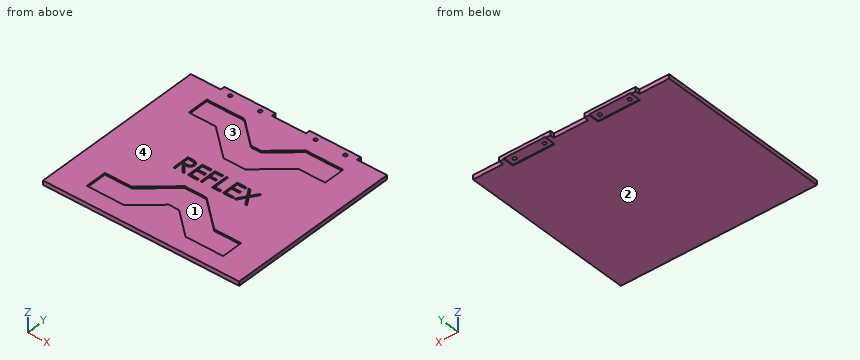
```python
from build123d import *

# Parameters (mm, degrees)
BOSS_EXTRU_1_DEPTH      = 5
ENL_V_MAT_EXTRU_2_DEPTH = 2
ENL_V_MAT_EXTRU_3_DEPTH = 2
ESQUISSE4_W             = 49
ESQUISSE4_H             = 12.519470299
ENL_V_MAT_EXTRU_5_DEPTH = 1
ESQUISSE5_R             = 2
ENL_V_MAT_EXTRU_6_DEPTH = 262.315639817


with BuildPart() as part:
    # Esquisse1 → Boss.-Extru.1 (new body)
    with BuildSketch(Plane.XY):
        Polygon((-56, 10.102941176), (-21, 10.102941176), (-21, 15.102941176), (39, 15.102941176), (39, 10.102941176), (79, 10.102941176), (79, 15.102941176), (139, 15.102941176), (139, 10.102941176), (174, 10.102941176), (174, -194.897058824), (-56, -194.897058824), align=None)
    extrude(amount=BOSS_EXTRU_1_DEPTH)

    # Esquisse2 → Enlèv. mat.-Extru.2 (cut)
    with BuildSketch(Plane.XY.offset(5)):
        Polygon((23.144921781, -9.214330656), (-20.950579999, -9.214330656), (-20.950579999, -34.214330656), (10.659241187, -34.214330656), (46.203012632, -65.443309996), (71.796987368, -65.443309996), (107.340758813, -34.214330656), (138.950579999, -34.214330656), (138.950579999, -9.214330656), (94.855078219, -9.214330656), (65.002138205, -35.443309996), (52.997861795, -35.443309996), align=None)
        Polygon((10.659241187, -150.579786991), (-20.950579999, -150.579786991), (-20.950579999, -175.579786991), (23.144921781, -175.579786991), (52.997861795, -149.350807651), (65.002138205, -149.350807651), (94.855078219, -175.579786991), (138.950579999, -175.579786991), (138.950579999, -150.579786991), (107.340758813, -150.579786991), (71.796987368, -119.350807651), (46.203012632, -119.350807651), align=None)
    extrude(amount=-ENL_V_MAT_EXTRU_2_DEPTH, mode=Mode.SUBTRACT)

    # Esquisse3 → Enlèv. mat.-Extru.3 (cut)
    # profile 1 of 6: a face of its own
    with BuildSketch(Plane.XY.offset(5)):
        with BuildLine():
            Line((20.856664396, -84.979311094), (24.859068242, -84.979311094))
            add(Edge.make_bspline(
                [(24.859068242, -84.979311094), (25.126160405, -84.980200157), (25.639006945, -84.981907256), (26.373711347, -84.991425901), (27.041294758, -85.018707934), (27.641408126, -85.042185554), (28.17404044, -85.084996647), (28.640824959, -85.125914631), (29.039611801, -85.179478407), (29.281016666, -85.229223681), (29.390318242, -85.251746992)],
                knots=[0, 0, 0, 0, 1.410062039, 2.707475311, 3.878576406, 4.937260626, 5.877586885, 6.699081471, 7.410979367, 8, 8, 8, 8], degree=3))
            add(Edge.make_bspline(
                [(29.390318242, -85.251746992), (29.536641809, -85.287899937), (29.826167463, -85.359434586), (30.243024983, -85.510632305), (30.640249692, -85.685601589), (31.016191545, -85.891108562), (31.368967495, -86.128678732), (31.702214985, -86.39421086), (32.017446204, -86.686252036), (32.301912662, -87.012165416), (32.570135815, -87.354088328), (32.796356538, -87.723824081), (32.991364993, -88.110461382), (33.14662509, -88.51793234), (33.271642082, -88.942285322), (33.359792021, -89.387364161), (33.41265595, -89.851141161), (33.418037982, -90.167472069), (33.42076696, -90.327868787)],
                knots=[0, 0, 0, 0, 1.027469482, 2.033020251, 3.019912614, 3.986113645, 4.951240523, 5.91722682, 6.890402269, 7.87763091, 8.8651537, 9.85103654, 10.82876324, 11.815024772, 12.821070561, 13.842952187, 14.906261191, 16, 16, 16, 16], degree=3))
            add(Edge.make_bspline(
                [(33.42076696, -90.327868787), (33.412372686, -90.594355099), (33.395993281, -91.114338915), (33.243278403, -91.868972523), (32.993126862, -92.572911464), (32.648422353, -93.225269395), (32.20945392, -93.813330226), (31.681883685, -94.329847113), (31.065417334, -94.762075185), (30.491535529, -95.061805498), (29.984597245, -95.253764975), (29.567264029, -95.388829883), (29.112024157, -95.493183971), (28.623239388, -95.586670438), (28.098875642, -95.657251549), (27.540189703, -95.708946374), (26.946783122, -95.741255224), (26.539131297, -95.74606668), (26.329420807, -95.748541864)],
                knots=[0, 0, 0, 0, 1.260483769, 2.459530307, 3.627416485, 4.787058657, 5.939039949, 7.08810263, 8.267026773, 9.491475466, 10.141966685, 10.831826277, 11.566392101, 12.351337768, 13.187381173, 14.07005841, 15.007169909, 16, 16, 16, 16], degree=3))
            Line((26.329420807, -95.748541864), (33.677177217, -104.979311094))
            Line((33.677177217, -104.979311094), (31.457625935, -104.979311094))
            Line((31.457625935, -104.979311094), (24.109869525, -95.748541864))
            Line((24.109869525, -95.748541864), (22.651536191, -95.748541864))
            Line((22.651536191, -95.748541864), (22.651536191, -104.979311094))
            Line((22.651536191, -104.979311094), (20.856664396, -104.979311094))
            Line((20.856664396, -104.979311094), (20.856664396, -84.979311094))
        make_face()
        with BuildLine():
            Line((22.651536191, -87.030593146), (22.651536191, -93.697259812))
            Line((22.651536191, -93.697259812), (26.313395166, -93.725304684))
            add(Edge.make_bspline(
                [(26.313395166, -93.725304684), (26.484366817, -93.725380322), (26.815758571, -93.72552693), (27.295190942, -93.702705352), (27.74159158, -93.676743533), (28.153253021, -93.637032987), (28.530359166, -93.585855434), (28.872721527, -93.521838382), (29.180898966, -93.447255167), (29.540319186, -93.331817305), (29.941670794, -93.148925772), (30.377850564, -92.882837208), (30.749292494, -92.548156527), (31.06310885, -92.165451064), (31.31527703, -91.744672499), (31.493060198, -91.290864675), (31.605874154, -90.815484115), (31.619180128, -90.48875207), (31.625895166, -90.323862376)],
                knots=[0, 0, 0, 0, 1.146690395, 2.22261258, 3.21895312, 4.145990853, 4.996080663, 5.770904154, 6.481378293, 7.121626537, 8.300444488, 9.431385265, 10.535395872, 11.636531494, 12.74115979, 13.810798291, 14.895190096, 16, 16, 16, 16], degree=3))
            add(Edge.make_bspline(
                [(31.625895166, -90.323862376), (31.619025902, -90.163024812), (31.605413529, -89.844303448), (31.494277709, -89.377698247), (31.306338387, -88.937315675), (31.053068456, -88.524947189), (30.744501856, -88.150628698), (30.382685783, -87.830359252), (29.977513239, -87.566076597), (29.598820677, -87.397194423), (29.260339463, -87.293652404), (28.966455692, -87.220788611), (28.634390105, -87.162248788), (28.262530341, -87.115345583), (27.852463879, -87.075031616), (27.402117302, -87.047878595), (26.914478557, -87.031799372), (26.576496094, -87.031004578), (26.401536191, -87.030593146)],
                knots=[0, 0, 0, 0, 1.101028733, 2.181837193, 3.264309656, 4.369019818, 5.486613113, 6.575447106, 7.666700264, 8.788928104, 9.402425223, 10.0903467, 10.862060571, 11.710948788, 12.657782767, 13.684531032, 14.801375019, 16, 16, 16, 16], degree=3))
            Line((26.401536191, -87.030593146), (22.651536191, -87.030593146))
        make_face(mode=Mode.SUBTRACT)
    # profile 2 of 6: a face of its own
    with BuildSketch(Plane.XY.offset(5)):
        Polygon((37.779741319, -84.979311094), (49.061792601, -84.979311094), (49.061792601, -87.030593146), (39.574613114, -87.030593146), (39.574613114, -93.184439299), (49.061792601, -93.184439299), (49.061792601, -95.235721351), (39.574613114, -95.235721351), (39.574613114, -102.928029043), (49.061792601, -102.928029043), (49.061792601, -104.979311094), (37.779741319, -104.979311094), align=None)
    # profile 3 of 6: a face of its own
    with BuildSketch(Plane.XY.offset(5)):
        Polygon((52.651536191, -84.979311094), (62.395125935, -84.979311094), (62.395125935, -87.030593146), (54.446407986, -87.030593146), (54.446407986, -93.184439299), (62.395125935, -93.184439299), (62.395125935, -95.235721351), (54.446407986, -95.235721351), (54.446407986, -104.979311094), (52.651536191, -104.979311094), align=None)
    # profile 4 of 6: a face of its own
    with BuildSketch(Plane.XY.offset(5)):
        Polygon((65.984869525, -84.979311094), (67.779741319, -84.979311094), (67.779741319, -102.928029043), (75.472049012, -102.928029043), (75.472049012, -104.979311094), (65.984869525, -104.979311094), align=None)
    # profile 5 of 6: a face of its own
    with BuildSketch(Plane.XY.offset(5)):
        Polygon((78.805382345, -84.979311094), (90.087433627, -84.979311094), (90.087433627, -87.030593146), (80.60025414, -87.030593146), (80.60025414, -93.184439299), (90.087433627, -93.184439299), (90.087433627, -95.235721351), (80.60025414, -95.235721351), (80.60025414, -102.928029043), (90.087433627, -102.928029043), (90.087433627, -104.979311094), (78.805382345, -104.979311094), align=None)
    # profile 6 of 6: a face of its own
    with BuildSketch(Plane.XY.offset(5)):
        Polygon((92.266920807, -84.979311094), (94.338234909, -84.979311094), (99.574613114, -93.160400838), (104.810991319, -84.979311094), (106.882305422, -84.979311094), (100.612273371, -94.778990582), (107.138715678, -104.979311094), (105.067401576, -104.979311094), (99.574613114, -96.397580325), (94.081824653, -104.979311094), (92.01051055, -104.979311094), (98.540959268, -94.778990582), align=None)
    extrude(amount=-ENL_V_MAT_EXTRU_3_DEPTH, mode=Mode.SUBTRACT)

    # Esquisse4 → Enlèv. mat.-Extru.5 (cut)
    with BuildSketch(Plane(origin=(0, 0, 0), x_dir=(-1, 0, 0), z_dir=(0, 0, -1))):
        with Locations((-9, 8.843206027)):
            Rectangle(ESQUISSE4_W, ESQUISSE4_H)
        with Locations((-109, 8.843206027)):
            Rectangle(ESQUISSE4_W, ESQUISSE4_H)
    extrude(amount=-ENL_V_MAT_EXTRU_5_DEPTH, mode=Mode.SUBTRACT)

    # Esquisse5 → Enlèv. mat.-Extru.6 (cut, through all)
    with BuildSketch(Plane(origin=(0, 0, 0), x_dir=(-1, 0, 0), z_dir=(0, 0, -1))):
        with Locations((8.5, 8.583470877)):
            Circle(ESQUISSE5_R)
        with Locations(Location((-26.5, 8.583470877, 0), (0, 0, 180))):
            Circle(ESQUISSE5_R)
        with Locations((-126.5, 8.583470877)):
            Circle(ESQUISSE5_R)
        with Locations((-91.5, 8.583470877)):
            Circle(ESQUISSE5_R)
    extrude(amount=-ENL_V_MAT_EXTRU_6_DEPTH, mode=Mode.SUBTRACT)


solid = part.part
```
The model under review builds one solid part; all positions refer to its coordinate system, in mm. Face numbers are marked on the shaded views. A direction names the side the tool comes from. Round coordinates to 2 decimals unless told otherwise and drop trailing zeros. Write each loop counter-clockwise with the first axis right and the second up, starting at its lowest first coordinate (ties: lowest second). Pieces come first, ordered by that corner, then holes.
(1) We need section A-A on x = 4. Give the boundary of the cut face in (y, z).
(2) We need section C-C on y = -134. Give the boundary of the cut face in (x, z), and give its area (3 significant figures).
(3) Insertion check: pin 1 (2 mm diameter, centred on x = 60.5, z = 4, fed in from +Y); pin 2 (2.5 mm diameter, centred on x = 126.5, y = 8.58, fed in from -Z). Each pin has a flat end and moves straight along its axis. Give the tip position at first contact, or say it passes through.
(4) Wall thickness on L1, parallel to Y at x = 126.5, z = 2.45; L2, parallel to Y at x = 69, z = 3.3; L3, parallel to Z at x = 31, y = -42.5: over which ranges is each line inside the solid? List them lowest first.
(5) Machinability: for the marked faces 3 and 4, which of the approach directions +Z, -Z, +X, -X, +Y, -Y give a long, thin tool a straight path to every point of the face, cutting with its end or side? Answer none if there is none.
(6) We need section D-D on y = -162. Give the boundary of the cut face in (x, z).
(7) We need section B-B on y = -31. Give the boundary of the cut face in (x, z), and give its area (3 significant figures).
(8) Mouldability with a two-part tool opening along X and no side actions: class the marked faces 1 and 2 as +X half, -X half, draft (parallel to the pull), parting line (faces both ways), or undercut.
Findings below:
1. outline: (-194.9, 0) - (2.58, 0) - (2.58, 1) - (15.1, 1) - (15.1, 5) - (-9.21, 5) - (-9.21, 3) - (-34.21, 3) - (-34.21, 5) - (-150.58, 5) - (-150.58, 3) - (-175.58, 3) - (-175.58, 5) - (-194.9, 5) - close
2. outline: (-56, 0) - (174, 0) - (174, 5) - (88.47, 5) - (88.47, 3) - (29.53, 3) - (29.53, 5) - (-56, 5) - close
2. area: 1,030 mm2
3. pin 1: stops at y = 10.1
3. pin 2: passes through
4. L1: y = -194.9 to 6.58, 10.58 to 15.1
4. L2: y = -194.9 to -152.86, -119.35 to -104.98, -102.93 to -65.44, -31.93 to 10.1
4. L3: z = 0 to 3
5. face 3: +Z
5. face 4: +Z, +X, -X, +Y, -Y
6. outline: (-56, 0) - (174, 0) - (174, 5) - (138.95, 5) - (138.95, 3) - (79.4, 3) - (79.4, 5) - (38.6, 5) - (38.6, 3) - (-20.95, 3) - (-20.95, 5) - (-56, 5) - close
7. outline: (-56, 0) - (174, 0) - (174, 5) - (138.95, 5) - (138.95, 3) - (70.06, 3) - (70.06, 5) - (47.94, 5) - (47.94, 3) - (-20.95, 3) - (-20.95, 5) - (-56, 5) - close
7. area: 874 mm2
8. face 1: undercut
8. face 2: draft
